Input: part model. Units: mm. Frame: model coordinates. Face numbers are marked on the shaded views. A direction names the side the tool comes from. Give positions to 0.01 mm unless a question says otherwise; leave off trailing zeros. Write each loop counter-clockwise with the first axis right and the second up, starting at its lowest first coordinate (ties: lowest second). Pieces come first, ordered by that corner, then holes. Notation, with made-up numbers: (11.5, 9.25) - (23.5, 9.25) arc R13 ccw to (23.5, 14.25) - close; hole circle Ø8 at (62.25, 2.5). An arc over 180 degrees is marked (long way). Answer as CSV lines item,"result". Start each with the question number.
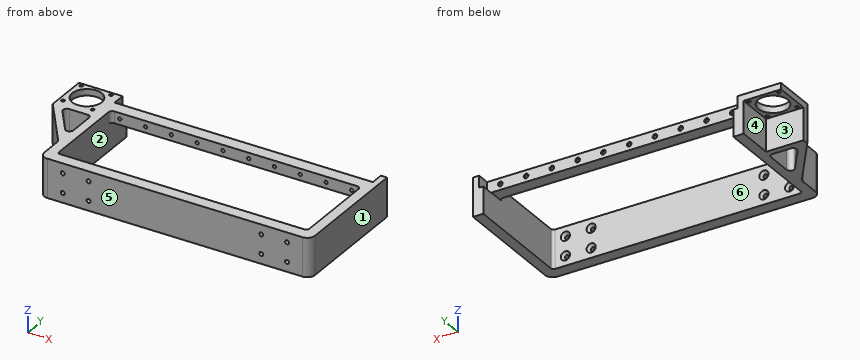
Autodesk Inventor part; units mm, degrees
ref_plane "YZ Plane" through (0, 0, 0) normal (1, 0, 0) x (0, 1, 0)
ref_plane "XZ Plane" through (0, 0, 0) normal (0, 1, 0) x (-1, 0, 0)
ref_plane "XY Plane" through (0, 0, 0) normal (0, 0, 1) x (1, 0, 0)
sketch "Sketch1" plane through (0, 0, 0) normal (0, 1, 0) x (-1, 0, 0)
  line L0 (96.4528, 98.5481) -> (-113.5472, 98.5481)
  line L1 (-113.5472, 98.5481) -> (-113.5472, 68.5481)
  line L2 (-113.5472, 68.5481) -> (96.4528, 68.5481)
  line L3 (96.4528, 68.5481) -> (96.4528, 98.5481)
  point P0 (0, 0)
  dimension "d0" = 210
  dimension "d1" = 30
extrude "Extrusion1" add sketch "Sketch1" along normal blind 9.5
sketch "Sketch2" plane through (0, 9.5, 0) normal (0, 1, 0) x (1, 0, 0)
  line L0 (-96.4528, -68.5481) -> (-96.4528, -98.5481)
  line L1 (-96.4528, -98.5481) -> (-88.4528, -98.5481)
  line L2 (-88.4528, -98.5481) -> (-88.4528, -68.5481)
  line L3 (-88.4528, -68.5481) -> (-96.4528, -68.5481)
  line L4 (-96.4528, -68.5481) -> (-96.4528, -98.5481)
  line L5 (113.5472, -98.5481) -> (113.5472, -68.5481)
  line L6 (113.5472, -98.5481) -> (105.5472, -98.5481)
  line L7 (105.5472, -98.5481) -> (105.5472, -68.5481)
  line L8 (105.5472, -68.5481) -> (113.5472, -68.5481)
  line L9 (113.5472, -68.5481) -> (113.5472, -98.5481)
  point P0 (0, 0)
  point P1 (-96.4528, -68.5481)
  point P2 (-96.4528, -68.5481)
  dimension "d4" = 8
  dimension "d5" = 8
  dimension "d6" = 30
extrude "Extrusion2" add sketch "Sketch2" along normal blind 87
sketch "Sketch3" plane through (0, 9.5, 0) normal (0, 1, 0) x (1, 0, 0)
  circle A0 centre (95.5472, -91.0481) radius 1.55
  circle A1 centre (95.5472, -76.0481) radius 1.55
  circle A2 centre (-78.4528, -76.0481) radius 1.55
  circle A3 centre (-78.4528, -91.0481) radius 1.55
  circle A4 centre (75.5472, -91.0481) radius 1.55
  circle A5 centre (75.5472, -76.0481) radius 1.55
  circle A6 centre (-58.4528, -91.0481) radius 1.55
  circle A7 centre (-58.4528, -76.0481) radius 1.55
  line L0 (-88.4528, -98.5481) -> (105.5472, -98.5481)
  line L1 (105.5472, -68.5481) -> (105.5472, -98.5481)
  line L2 (-88.4528, -98.5481) -> (-88.4528, -68.5481)
  point P0 (0, 0)
  dimension "d9" = 3.1
  dimension "d10" = 3.1
  dimension "d11" = 3.1
  dimension "d12" = 3.1
  dimension "d13" = 3.1
  dimension "d14" = 3.1
  dimension "d15" = 3.1
  dimension "d16" = 3.1
  dimension "d17" = 20
  dimension "d18" = 15
  dimension "d19" = 20
  dimension "d20" = 15
  dimension "d21" = 7.5
  dimension "d22" = 7.5
  dimension "d23" = 10
  dimension "d24" = 10
  dimension "d25" = 7.5
  dimension "d26" = 7.5
  dimension "d27" = 10
  dimension "d28" = 10
  dimension "d29" = 15
  dimension "d30" = 20
  dimension "d31" = 15
  dimension "d32" = 20
extrude "Extrusion3" cut sketch "Sketch3" against normal through all
chamfer "Chamfer1" distance 2 angle 45 8 edges at (93.9972, 9.5, 91.0481) (93.9972, 9.5, 76.0481) (73.9972, 9.5, 76.0481) (73.9972, 9.5, 91.0481) (-60.0028, 9.5, 91.0481) (-80.0028, 9.5, 91.0481) (-80.0028, 9.5, 76.0481) (-60.0028, 9.5, 76.0481)
fillet "Fillet1" radius 2 2 edges at (105.5472, 9.5, 83.5481) (-88.4528, 9.5, 83.5481)
fillet "Fillet2" radius 6 2 edges at (113.5472, 0, 83.5481) (-96.4528, 0, 83.5481)
sketch "Sketch4" plane through (-86.4528, 9.5, 98.5481) normal (0, 0, 1) x (1, 0, 0)
  line L0 (-2, 2) -> (-2, 87)
  line L1 (192, 2) -> (192, 87)
  line L2 (-2, 77) -> (192, 77)
  line L3 (192, 77) -> (192, 67)
  line L4 (192, 67) -> (-2, 67)
  line L5 (-2, 67) -> (-2, 77)
  line L6 (-10, 87) -> (-2, 87)
  point P0 (86.4528, -9.5)
  point P1 (-2, 67)
  point P2 (192, 77)
  dimension "d40" = 10
  dimension "d41" = 10
extrude "Extrusion4" add sketch "Sketch4" against normal blind 9
sketch "Sketch5" plane through (0, 96.5, 0) normal (0, 1, 0) x (1, 0, 0)
  line L0 (105.5472, -98.5481) -> (105.5472, -68.5481)
  line L1 (105.5472, -98.5481) -> (108.7472, -98.5481)
  line L2 (108.7472, -98.5481) -> (108.7472, -89.3481)
  line L3 (108.7472, -89.3481) -> (105.5472, -89.3481)
  line L4 (105.5472, -89.3481) -> (105.5472, -98.5481)
  line L5 (-88.4528, -98.5481) -> (-88.4528, -68.5481)
  line L6 (-88.4528, -98.5481) -> (-91.6528, -98.5481)
  line L7 (-91.6528, -98.5481) -> (-91.6528, -89.3481)
  line L8 (-91.6528, -89.3481) -> (-88.4528, -89.3481)
  line L9 (-88.4528, -89.3481) -> (-88.4528, -98.5481)
  point P0 (0, 0)
  dimension "d44" = 3.2
  dimension "d45" = 9.2
  dimension "d46" = 3.2
  dimension "d47" = 9.2
extrude "Extrusion5" cut sketch "Sketch5" against normal up to surface (10 mm away)
sketch "Sketch6" plane through (-88.4528, 86.5, 89.5481) normal (0, 1, 0) x (1, 0, 0)
  circle A0 centre (187, -4.5) radius 1.3
  line L0 (197.2, -9) -> (-3.2, -9)
  line L1 (197.2, 0.2) -> (197.2, -9)
  circle A1 centre (167, -4.5) radius 1.3
  circle A2 centre (147, -4.5) radius 1.3
  circle A3 centre (127, -4.5) radius 1.3
  circle A4 centre (107, -4.5) radius 1.3
  circle A5 centre (87, -4.5) radius 1.3
  circle A6 centre (67, -4.5) radius 1.3
  circle A7 centre (47, -4.5) radius 1.3
  circle A8 centre (27, -4.5) radius 1.3
  circle A9 centre (7, -4.5) radius 1.3
  point P0 (88.4528, 89.5481)
  dimension "d50" = 2.6
  dimension "d51" = 4.5
  dimension "d52" = 10.2
  dimension "d55" = 20
extrude "Extrusion6" cut sketch "Sketch6" against normal up to surface (10 mm away)
chamfer "Chamfer2" distance 0.5 angle 45 10 edges at (97.2472, 86.5, 94.0481) (77.2472, 86.5, 94.0481) (57.2472, 86.5, 94.0481) (37.2472, 86.5, 94.0481) (17.2472, 86.5, 94.0481) (-2.7528, 86.5, 94.0481) (-22.7528, 86.5, 94.0481) (-42.7528, 86.5, 94.0481) (-62.7528, 86.5, 94.0481) (-82.7528, 86.5, 94.0481)
sketch "Sketch7" plane through (-96.4528, 96.5, 68.5481) normal (-1, 0, 0) x (0, 0, 1)
  line L0 (0, 0) -> (30, 0)
  line L1 (30, 0) -> (25, 0)
  line L2 (25, 0) -> (25, -33)
  line L3 (25, -33) -> (30, -33)
  line L4 (30, -33) -> (30, 0)
  point P0 (-68.5481, -96.5)
  dimension "d65" = 5
  dimension "d66" = 33
extrude "Extrusion7" add sketch "Sketch7" along normal blind 29
sketch "Sketch8" plane through (-96.4528, 6, 68.5481) normal (-1, 0, 0) x (0, 0, 1)
  line L0 (30, 57.5) -> (25, 57.5)
  line L1 (0, 5.5) -> (0, 90.5)
  line L2 (25, 57.5) -> (0, 57.5)
  line L3 (0, 57.5) -> (0, 62.3)
  line L4 (0, 62.3) -> (25, 62.3)
  line L5 (25, 62.3) -> (25, 57.5)
  point P0 (-68.5481, -6)
  point P1 (0, 57.5)
  dimension "d69" = 4.8
extrude "Extrusion8" add sketch "Sketch8" along normal blind 29
sketch "Sketch9" plane through (-96.4528, 96.5, 93.5481) normal (0, 0, -1) x (-1, 0, 0)
  circle A0 centre (14.1, -14.1) radius 11.5
  line L0 (0, -28.2) -> (29, -28.2)
  line L1 (0, -28.2) -> (0, 0)
  point P0 (-96.4528, -96.5)
  dimension "d40" = 10
  dimension "d72" = 23
  dimension "d73" = 14.1
  dimension "d74" = 14.1
extrude "Extrusion9" cut sketch "Sketch9" against normal through all
fillet "Fillet4" radius 3 2 edges at (105.5472, 76.5, 94.0481) (-88.4528, 76.5, 94.0481)
sketch "Sketch10" plane through (103.5472, 9.5, 68.5481) normal (0, 0, -1) x (-1, 0, 0)
  line L0 (200, 54) -> (229, 54)
  line L1 (200, 54) -> (229, 54)
  line L2 (229, 54) -> (200, 14)
  line L3 (200, -3.5) -> (200, 54)
  line L4 (200, 54) -> (200, 14)
  point P0 (103.5472, -9.5)
  dimension "d79" = 40
extrude "Extrusion10" add sketch "Sketch10" against normal up to surface (30 mm away)
sketch "Sketch11" plane through (103.5472, 9.5, 68.5481) normal (0, 0, -1) x (-1, 0, 0)
  line L0 (222, 54) -> (199, 54)
  line L1 (199, 54) -> (199, 22.2759)
  line L2 (199, 22.2759) -> (222, 54)
  line L3 (200, 58.8) -> (229, 58.8)
  line L4 (192, 2) -> (192, 87)
  line L5 (200, 14) -> (229, 54)
  point P0 (103.5472, -9.5)
  dimension "d82" = 4.8
  dimension "d83" = 7
  dimension "d85" = 23
extrude "Extrusion11" cut sketch "Sketch11" against normal through all
fillet "Fillet5" radius 3 3 edges at (-95.4528, 63.5, 83.5481) (-95.4528, 31.7759, 83.5481) (-118.4528, 63.5, 83.5481)
fillet "Fillet6" radius 6 1 edges at (-96.4528, 23.5, 83.5481)
sketch "Sketch12" plane through (-90.4528, 0, 98.5481) normal (0, 0, 1) x (1, 0, 0)
  circle A0 centre (-31.6, 93.9) radius 1.3
  circle A1 centre (-8.6, 93.9) radius 1.3
  circle A2 centre (-8.6, 70.9) radius 1.3
  circle A3 centre (-31.6, 70.9) radius 1.3
  circle A4 centre (-20.1, 82.4) radius 11.5
  point P0 (90.4528, 0)
  dimension "d90" = 2.6
  dimension "d91" = 2.6
  dimension "d92" = 2.6
  dimension "d93" = 2.6
  dimension "d94" = 11.5
  dimension "d95" = 11.5
  dimension "d96" = 11.5
  dimension "d97" = 11.5
  dimension "d98" = 11.5
  dimension "d99" = 11.5
  dimension "d100" = 11.5
  dimension "d101" = 11.5
extrude "Extrusion12" cut sketch "Sketch12" against normal through all contours A0 | A1 | A2 | A3
properties part number "gantry_R"
1) Reachability of the marked faces 4, 5 and 6 from +Z, -Z, +X, -X, +Y, -Y: full face, straight path, thin tool, end or side. Return the list, or none.
2) Contact query for flat-ended pins moving along their axis: P1, Ø7.5, axis at x = -112.5, z = 87, coming from the +Y side; P2, Ø2, axis at y = 42.5, z = 82, coming from the -X side; P3, Ø12, axis at x = 59.5, z = 86, coming from the +Y side; P4, Ø1.9, axis at x = 75.55, z = 76.05, coming from the -Y side. Output: stop coordinate, or through.
3) Pull-direction query (X, two-part tool) for the marked faces 1, 2 and 3; classes: +X half, -X half, draft (parallel to the pull), parting line (faces both ways), or undercut.
4) Cut plane B-B on y = 82.4. State how many separate pieces and enclosed holes the cut face has, and give its area (3 significant figures).
5) Material intervals for line 1 (Y direction, x = -11, z = 92.5); line 2 (X direction, y = 62, z = 81); line 3 (X direction, y = 21.5, z = 91.5), sorted ascending. Write a range as from..to.
6) Cut plane A-A on x = 85. Output: boundary loops of the cut face in (y, z).
Numbers:
1,face 4,"-Z, -X, +Y"
1,face 5,"+Z, -Z, +X, -X, -Y"
1,face 6,"+Z, -Z"
2,P1,"stops at y = 68.3"
2,P2,"stops at x = -110.95"
2,P3,"stops at y = 86.5"
2,P4,"passes through"
3,face 1,"+X half"
3,face 2,"undercut"
3,face 3,"draft"
4,separate pieces,"2"
4,enclosed holes,"10"
4,area,"2,200 mm²"
5,line 1,"y = 0..9.5, 76.5..86.5"
5,line 2,"x = -124.37..-115.17, -95.85..-88.45, 105.55..113.55"
5,line 3,"x = -96.45..-88.45, 105.55..113.55"
6,outline,"(0, 68.55) - (9.5, 68.55) - (9.5, 98.55) - (0, 98.55) - close; (76.5, 89.55) - (86.5, 89.55) - (86.5, 98.55) - (76.5, 98.55) - close"
